The figure shows three views and two pictorial views of one solid part (mm, origin at its lowest corner). Answer the questions. A direction names the side the tool comes from. Round coordinates to 2 decimals unless told otherwise and drop trailing zeros. Order: outer loops, then holes, each group sorted by start corner. A loop starts at its lowest first (then second) coordinate and runs counter-clockwise, first axis right, second up. Notation, with made-up numbers: (-6, 25) - (52, 25) arc R22 ccw to (52, 50) - close; hole circle Ø2 at (7, 82.5). An arc over 180 degrees is marked (long way). Answer as a JSON object with one key per item and string values. Group by question number.
Q1. A tool of negligible diameter and unlimited length cuts with its end or side. For the marked faces 1 and 2, from which of +Z, -Z, +X, -X, +Y, -Y can it reach the whole face along a straight path? Write none if from no direction.
Q2. A cutting plane is placed at A-A on y = 60. Determine the outline of the cut face in (x, z), and give its area (3 significant figures).
Q3. A cutting plane is placed at C-C on z = 38.5. Determine the outline of the cut face in (x, y) (3 decimals), and give its area (3 significant figures).
Q4. A cutting plane is placed at B-B on x = 118.9. Determine the outline of the cut face in (y, z) (3 decimals), and give its area (3 significant figures).
Q5. Consider line 1 (X direction, y = 100, z = 38.5) (3 decimals); line 2 (X direction, y = 99, z = 38); line 3 (Z direction, x = 58, y = 98). Determine where each line is inside the solid, lowest interval first.
Q6. Given pin 1 Ø4 at (x, z) = (65, 28.5) entering from -Y; pin 2 Ø6 at (x, y) = (130.5, 29.5) entering from -Z, each flat-ended and moving along its own axis, determine where each tip first touches the part or whether it passes through.
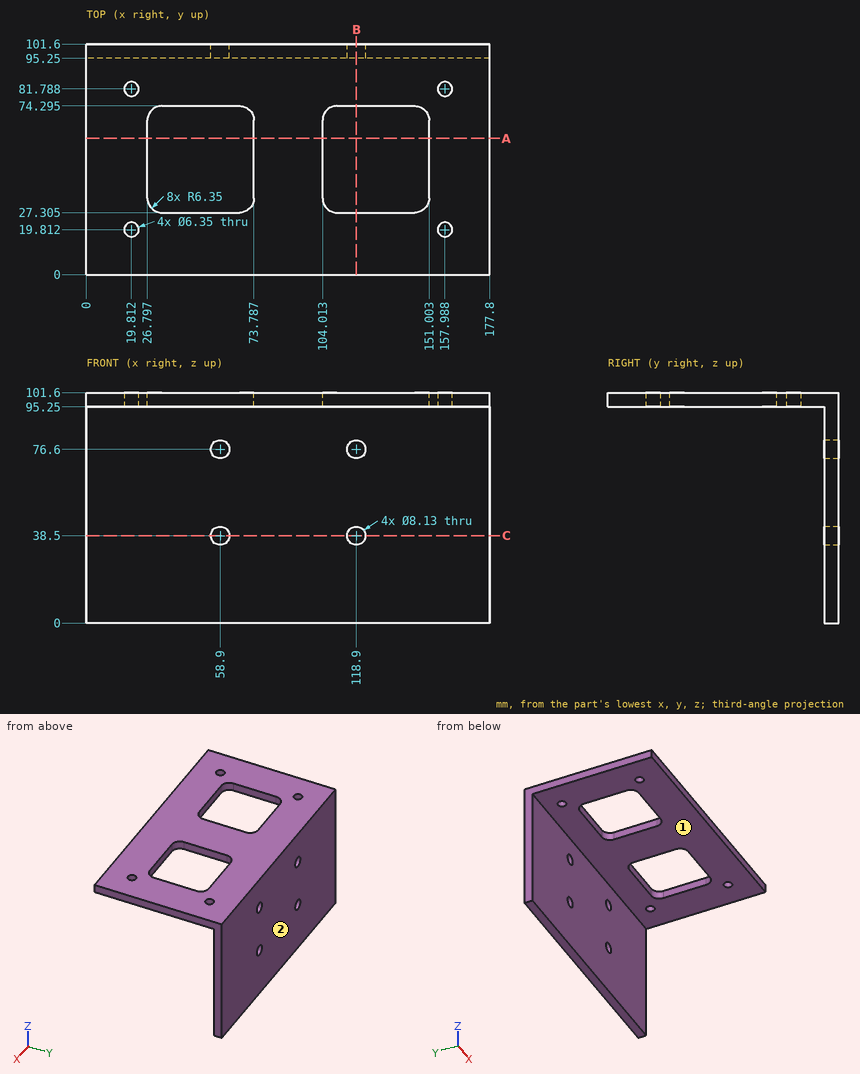
Result set:
{
 "1": {"face 1": "-Z, +X, -X, -Y", "face 2": "+Z, -Z, +X, -X, +Y"},
 "2": {"outline": "(0, 95.25) - (26.8, 95.25) - (26.8, 101.6) - (0, 101.6) - close; (73.79, 95.25) - (104.01, 95.25) - (104.01, 101.6) - (73.79, 101.6) - close; (151, 95.25) - (177.8, 95.25) - (177.8, 101.6) - (151, 101.6) - close", "area": "532 mm²"},
 "3": {"outline": "(0, 95.25) - (54.835, 95.25) - (54.835, 101.6) - (0, 101.6) - close; (62.965, 95.25) - (114.835, 95.25) - (114.835, 101.6) - (62.965, 101.6) - close; (122.965, 95.25) - (177.8, 95.25) - (177.8, 101.6) - (122.965, 101.6) - close", "area": "1,030 mm²"},
 "4": {"outline": "(0, 95.25) - (27.305, 95.25) - (27.305, 101.6) - (0, 101.6) - close; (74.295, 95.25) - (95.25, 95.25) - (95.25, 80.665) - (101.6, 80.665) - (101.6, 101.6) - (74.295, 101.6) - close; (95.25, 0) - (101.6, 0) - (101.6, 34.435) - (95.25, 34.435) - close; (95.25, 42.565) - (101.6, 42.565) - (101.6, 72.535) - (95.25, 72.535) - close", "area": "848 mm²"},
 "5": {"line 1": "x = 0 to 54.835, 62.965 to 114.835, 122.965 to 177.8", "line 2": "x = 0 to 54.87, 62.93 to 114.87, 122.93 to 177.8", "line 3": "z = 0 to 34.54, 42.46 to 72.64, 80.56 to 101.6"},
 "6": {"pin 1": "stops at y = 95.25", "pin 2": "stops at z = 95.25"}
}
